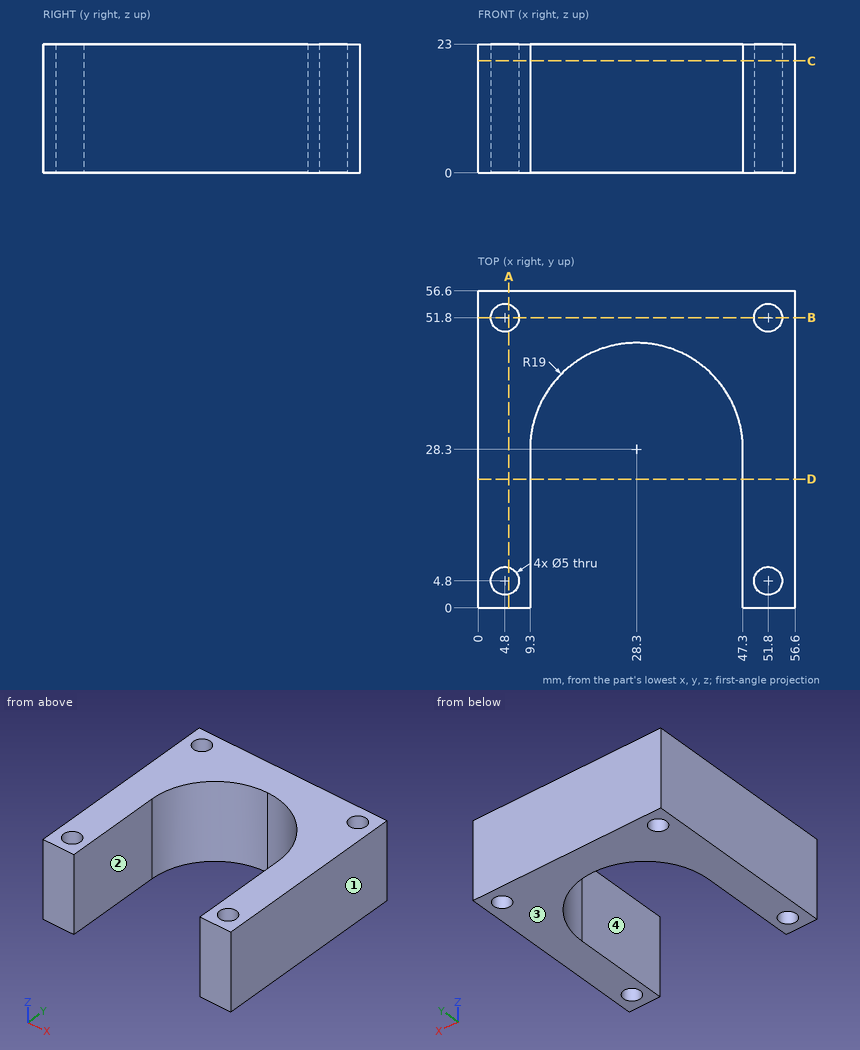
Part print with two shaded views. Sizes in mm from the minimum x, y, z corner. Coordinates: 2 decimals unless noted, no trailing zeros. Write each loop counter-clockwise with the first axis right and the second up, starting at its lowest first coordinate (ties: lowest second). Pieces come first, ordered by that corner, then holes. Notation, with made-up numbers: (25, 75) - (37, 75) arc R9 cw to (37, 80) - close; hole circle Ø10 at (29, 87.5). An arc over 180 degrees is marked (long way). Use a Markdown table: item, result. Add a question column.
Item 1: Drill centre lines: line 1 along Y through (x, z) = (51.8, 16.5); line 2 along X through (y, z) = (21, 17.5); line 3 along Y through (x, z) = (6.5, 16.5). Where is each one in solid material? Low to high.
Item 2: Band-saw the part on D-D, the plane y = 23. Write the cut outline in (x, z).
Item 3: Band-saw the part on B-B, the plane y = 51.8. Write the cut outline in (x, z).
Item 4: Band-saw the part on C-C, the plane z = 20. Write the cut outline in (x, y).
Item 5: Two-plate mould, pull along X, no slides. Class the marked faces 1, 2, 3 and 4: pulls with the +X half, pulls with the -X half, needs draft (parallel to the pull), parting line crosses it, or undercut.
Item 6: Drop flat-ended pins along their axis: pin 1 (1 mm diameter, centred on x = 26.5, z = 8.5, fed in from -Y); pin 2 (4 mm diameter, centred on x = 43, z = 2.5, fed in from -Y); pin 3 (2 mm diameter, centred on x = 38, z = 4.5, fed in from -Y). Give the stop position or say it passes through.
Item 7: Band-saw the part on A-A, the plane x = 5.5. Write the cut outline in (y, z).
A:
| question | item | result |
|---|---|---|
| 1 | line 1 | y = 0 to 2.3, 7.3 to 49.3, 54.3 to 56.6 |
| 1 | line 2 | x = 0 to 9.3, 47.3 to 56.6 |
| 1 | line 3 | y = 0 to 2.97, 6.63 to 49.97, 53.63 to 56.6 |
| 2 | outline | (0, 0) - (9.3, 0) - (9.3, 23) - (0, 23) - close; (47.3, 0) - (56.6, 0) - (56.6, 23) - (47.3, 23) - close |
| 3 | outline | (0, 0) - (2.3, 0) - (2.3, 23) - (0, 23) - close; (7.3, 0) - (49.3, 0) - (49.3, 23) - (7.3, 23) - close; (54.3, 0) - (56.6, 0) - (56.6, 23) - (54.3, 23) - close |
| 4 | outline | (0, 0) - (9.3, 0) - (9.3, 28.3) arc R19 cw to (47.3, 28.3) - (47.3, 0) - (56.6, 0) - (56.6, 56.6) - (0, 56.6) - close; hole circle Ø5 at (4.8, 4.8); hole circle Ø5 at (4.8, 51.8); hole circle Ø5 at (51.8, 4.8); hole circle Ø5 at (51.8, 51.8) |
| 5 | face 1 | pulls with the +X half |
| 5 | face 2 | undercut |
| 5 | face 3 | needs draft |
| 5 | face 4 | undercut |
| 6 | pin 1 | stops at y = 47.16 |
| 6 | pin 2 | stops at y = 37.36 |
| 6 | pin 3 | stops at y = 44 |
| 7 | outline | (0, 0) - (2.4, 0) - (2.4, 23) - (0, 23) - close; (7.2, 0) - (49.4, 0) - (49.4, 23) - (7.2, 23) - close; (54.2, 0) - (56.6, 0) - (56.6, 23) - (54.2, 23) - close |
